from build123d import *

# Parameters (mm, degrees)
F0_R     = 36
F0_R_2   = 1.5
F1_DEPTH = 3
F2_R     = 2
F3_R     = 5.08
F4_COUNT = 5


with BuildPart() as f1:
    # F0 (on Front) → F1 (new body)
    with BuildSketch(Plane.XZ):
        Circle(F0_R)
        with BuildLine():
            ThreePointArc((-0.9998699187, 30.9838709677), (0, 31), (0.9998699187, 30.9838709677))
            ThreePointArc((0.9998699187, 30.9838709677), (22.2710121849, 21.5639054037), (31, 0))
            ThreePointArc((31, 0), (-21.5639054037, -22.2710121849), (-0.9998699187, 30.9838709677))
        make_face(mode=Mode.SUBTRACT)
        with BuildLine():
            ThreePointArc((-1.5, 4.2426406871), (0, 4.5), (1.5, 4.2426406871))
            Line((1.5, 4.2426406871), (0.9998699187, 30.9838709677))
            ThreePointArc((0.9998699187, 30.9838709677), (0, 31), (-0.9998699187, 30.9838709677))
            Line((-0.9998699187, 30.9838709677), (-1.5, 4.2426406871))
        make_face()
        with BuildLine():
            ThreePointArc((-1.5, 4.2426406871), (-2.5980762114, -3.6742346142), (4.5, 0))
            ThreePointArc((4.5, 0), (3.6742346142, 2.5980762114), (1.5, 4.2426406871))
            ThreePointArc((1.5, 4.2426406871), (0, 4.5), (-1.5, 4.2426406871))
        make_face()
        Circle(F0_R_2, mode=Mode.SUBTRACT)
    extrude(amount=F1_DEPTH)

    # F2
    f2_edges = [f1.edges().sort_by_distance(p)[0] for p in [
        (0.99987, -1.5, 30.983871),
        (-0.99987, -1.5, 30.983871),
    ]]
    fillet(f2_edges, radius=F2_R)

    # F3
    f3_edges = [f1.edges().sort_by_distance(p)[0] for p in [
        (-1.5, -1.5, 4.242641),
        (1.5, -1.5, 4.242641),
    ]]
    fillet(f3_edges, radius=F3_R)

    # F4: F1 ×5 about axis
    f4_axis = Axis((0, 0, 0), (0, 1, 0))


with BuildPart() as f1_1:
    add(f1.part)
    for i in range(1, F4_COUNT):
        add(f1.part.rotate(f4_axis, i * 360 / F4_COUNT))


solid = f1_1.part
Here's how the part is built. I have some questions about the finished solid (model axes, mm). Give positions to 0.01 mm unless a question says otherwise; leave off trailing zeros. Order: outer loops, then holes, each group sorted by start corner. A loop starts at its lowest first (then second) coordinate and runs counter-clockwise, first axis right, second up. Notation, with made-up numbers: M 73.25,53 L 130.25,53 A10 cw 130.25,57 Z; hole C 18,74 d1. An arc over 180 degrees is marked long. Answer as a JSON object with one key per item and string values. Group by question number.
1) Suppose I cut it at B-B, the plane z = -8.5. Write out the boundary of the cut face in (x, y), plus the area to 3 significant figures.
2) Suppose I cut it at A-A, the plane z = 20. Write out the boundary of the cut face in (x, y).
3) Suppose I cut it at D-D, the plane y = -0.8. Count the separate pieces of the cut face and the enclosed holes in it, plus the area to 3 significant figures.
4) I'm going to push flat-ended pins straight in: pin 1 Ø1.5 at (x, y) = (0, -1) entering from -Z; pin 2 Ø2.5 at (x, z) = (0, 0) entering from -Y. Where does each tip first touch, or does it pass through?
5) We'd pull the mould along Z, two halves only. Please class faces 1 (the cylindrical face through (-28.32, -1.52, 11)), 2 (the cylindrical face through (-4.686, -1.479, 35.694)), 3 (the cylindrical face through (-1.706, -1.521, 30.33)): pulls with the +Z half, pulls with the -Z half, needs draft (parallel to the pull), parting line crosses it, or undercut.
6) Suppose I cut it at C-C, the plane x = 19. Write out the boundary of the cut face in (y, z).
7) Please list where these lines run through material, in increasing order: L1, parallel to Z at x = 0, y = -1.25; L2, parallel to Z at x = 5.5, y = -1.25; L3, parallel to Z at x = -19.5, y = -1.25. Write a range as [from, to].
Results found:
{
 "1": {"outline": "M -34.98,-3 L -29.81,-3 L -29.81,0 L -34.98,0 Z; M -7.86,-3 L -4.44,-3 L -4.44,0 L -7.86,0 Z; M 4.44,-3 L 7.86,-3 L 7.86,0 L 4.44,0 Z; M 29.81,-3 L 34.98,-3 L 34.98,0 L 29.81,0 Z", "area": "51.5 mm²"},
 "2": {"outline": "M -29.93,-3 L -23.69,-3 L -23.69,0 L -29.93,0 Z; M -1.21,-3 L 1.21,-3 L 1.21,0 L -1.21,0 Z; M 23.69,-3 L 29.93,-3 L 29.93,0 L 23.69,0 Z"},
 "3": {"separate pieces": "1", "enclosed holes": "6", "area": "1,460 mm²"},
 "4": {"pin 1": "z = -36", "pin 2": "through"},
 "5": {"face 1": "undercut", "face 2": "parting line crosses it", "face 3": "undercut"},
 "6": {"outline": "M -3,-30.58 L 0,-30.58 L 0,-23.5 L -3,-23.5 Z; M -3,4.9 L 0,4.9 L 0,7.43 L -3,7.43 Z; M -3,24.49 L 0,24.49 L 0,30.58 L -3,30.58 Z"},
 "7": {"L1": "[-36, -31], [-4.56, -1.5], [1.5, 36]", "L2": "[-35.58, -30.51], [-9.9, -5.12], [-0.09, 3.37], [30.51, 35.58]", "L3": "[-30.26, -23.54], [5.07, 7.59], [24.1, 30.26]"}
}
